Verification items for this drawing (mm, ordinates from the low corner). A direction names the side the tool comes from. Coordinates: 2 decimals unless noted, no trailing zeros. Write each loop counter-clockwise with the first axis right and the second up, starting at its lowest first coordinate (ties: lowest second). Pieces come first, ordered by that corner, then holes.
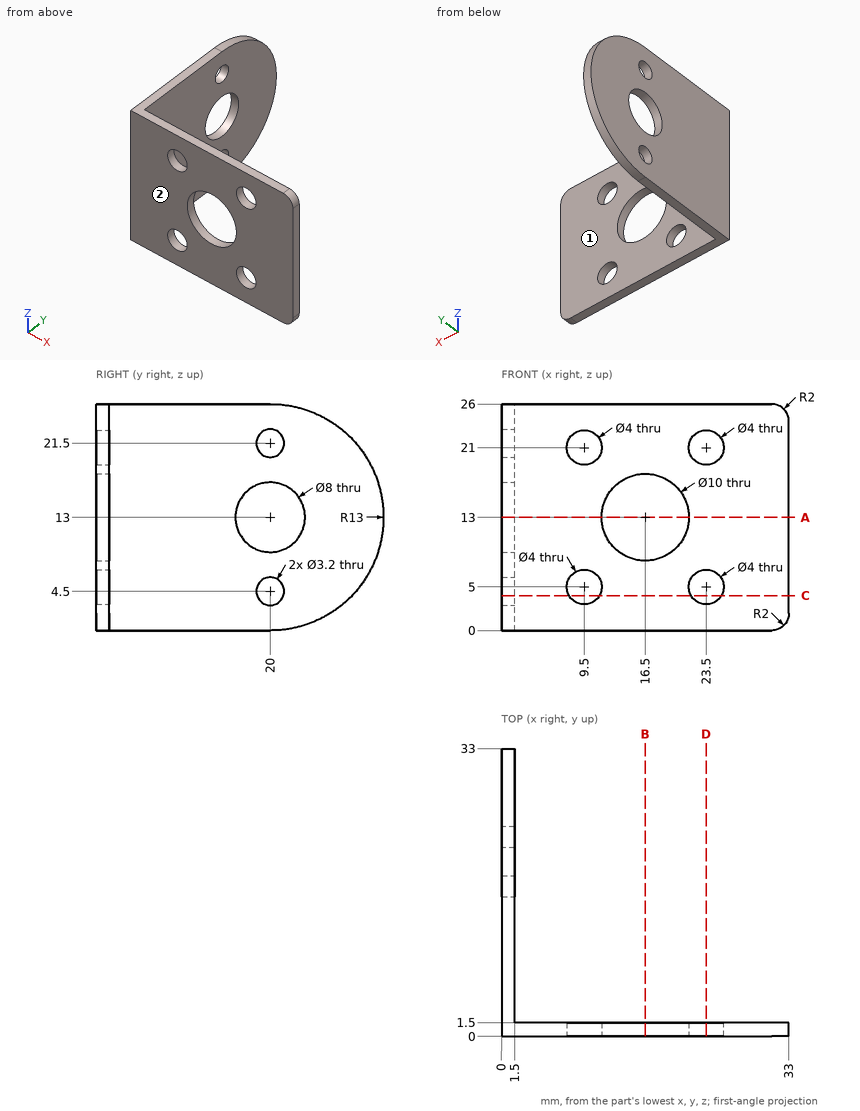
1. Gauge pin test, flat ends, axial feed: pin 1 Ø5 at (x, z) = (6, 23) entering from +Y; pin 2 Ø13 at (y, z) = (20, 13) entering from +X. Record the tip position at first contact, or that the pin passes through.
Computed values:
pin 1: stops at y = 1.5
pin 2: stops at x = 1.5
2. Access from +Z, -Z, +X, -X, +Y, -Y to the whole of each face (thin tool, end or side, straight path). Record for the marked faces 1 and 2.
Computed values:
face 1: +Z, -Z, +X, +Y
face 2: +Z, -Z, +X, -X, -Y
3. Sectioned sample at A-A, the plane z = 13. Record the boundary of the cut face in (x, y), and give its area (4 significant figures).
Computed values:
outline: (0, 0) - (11.5, 0) - (11.5, 1.5) - (1.5, 1.5) - (1.5, 16) - (0, 16) - close; (0, 24) - (1.5, 24) - (1.5, 33) - (0, 33) - close; (21.5, 0) - (33, 0) - (33, 1.5) - (21.5, 1.5) - close
area: 69.75 mm2
4. Thickness scan on line 1 along Z through (x, y) = (0.7, 20); line 2 along Z through (x, y) = (23.5, 0.7); line 3 along X through (y, z) = (18, 8.75). Record the ranges inside material, lowest first.
Computed values:
line 1: z = 0 to 2.9, 6.1 to 9, 17 to 19.9, 23.1 to 26
line 2: z = 0 to 3, 7 to 19, 23 to 26
line 3: x = 0 to 1.5
5. Sectioned sample at D-D, the plane x = 23.5. Record the boundary of the cut face in (y, z), and give its area (3 significant figures).
Computed values:
outline: (0, 0) - (1.5, 0) - (1.5, 3) - (0, 3) - close; (0, 7) - (1.5, 7) - (1.5, 19) - (0, 19) - close; (0, 23) - (1.5, 23) - (1.5, 26) - (0, 26) - close
area: 27.0 mm2
6. Sectioned sample at C-C, the plane z = 4. Record the boundary of the cut face in (x, y), and give its area (3 significant figures).
Computed values:
outline: (0, 0) - (7.77, 0) - (7.77, 1.5) - (1.5, 1.5) - (1.5, 18.48) - (0, 18.48) - close; (0, 21.52) - (1.5, 21.52) - (1.5, 29.38) - (0, 29.38) - close; (11.23, 0) - (21.77, 0) - (21.77, 1.5) - (11.23, 1.5) - close; (25.23, 0) - (33, 0) - (33, 1.5) - (25.23, 1.5) - close
area: 76.4 mm2
7. Sectioned sample at B-B, the plane x = 16.5. Record the boundary of the cut face in (y, z), and give its area (3 significant figures).
Computed values:
outline: (0, 0) - (1.5, 0) - (1.5, 8) - (0, 8) - close; (0, 18) - (1.5, 18) - (1.5, 26) - (0, 26) - close
area: 24.0 mm2
